Work out the finished part from the listing and answer in its coordinate system (mm). Face numbers are marked on the shaded views. A direction names the side the tool comes from. Coordinates: 2 decimals unless noted, no trailing zeros. Order: outer loops, then holes, each group sorted by start corner. A loop starts at its lowest first (then second) coordinate and runs counter-clockwise, first axis right, second up. Notation, with made-up numbers: M 83,-1 L 97,-1 A19 cw 97,20 Z; hole C -17,-30.5 d11. An arc over 180 degrees is marked long. Use a Markdown table: item, result.
from build123d import *

# Parameters (mm, degrees)
F0_R     = 0.5
F1_DEPTH = 75
F2_DEPTH = 58


with BuildPart() as f1:
    # F0 (on Front) → F1 (new body)
    with BuildSketch(Plane.XZ):
        with BuildLine():
            ThreePointArc((0.820651, 1.615282), (0.216927, 0.905898), (0, 0))
            ThreePointArc((0, 0), (2, -2), (4, 0))
            ThreePointArc((4, 0), (2.905898, 1.783073), (0.820651, 1.615282))
        make_face()
        with Locations((2, 0)):
            Circle(F0_R, mode=Mode.SUBTRACT)
    extrude(amount=F1_DEPTH)

    # F0 (on Front) → F2 (join)
    with BuildSketch(Plane.XZ):
        with BuildLine():
            Line((0, 9.6), (0, 0))
            ThreePointArc((0, 0), (0.216927, 0.905898), (0.820651, 1.615282))
            Line((0.820651, 1.615282), (0.820651, 10.211033))
            Line((0.820651, 10.211033), (-5.284584, 16.147118))
            Line((-5.284584, 16.147118), (-9.5, 16.147118))
            Line((-9.5, 16.147118), (-9.5, 15.5))
            Line((-9.5, 15.5), (-6.118823, 15.5))
            Line((-6.118823, 15.5), (0, 9.6))
        make_face()
        with BuildLine():
            ThreePointArc((0.820651, 1.615282), (0.216927, 0.905898), (0, 0))
            ThreePointArc((0, 0), (2, -2), (4, 0))
            ThreePointArc((4, 0), (2.905898, 1.783073), (0.820651, 1.615282))
        make_face()
        with Locations((2, 0)):
            Circle(F0_R, mode=Mode.SUBTRACT)
    extrude(amount=F2_DEPTH)


solid = f1.part
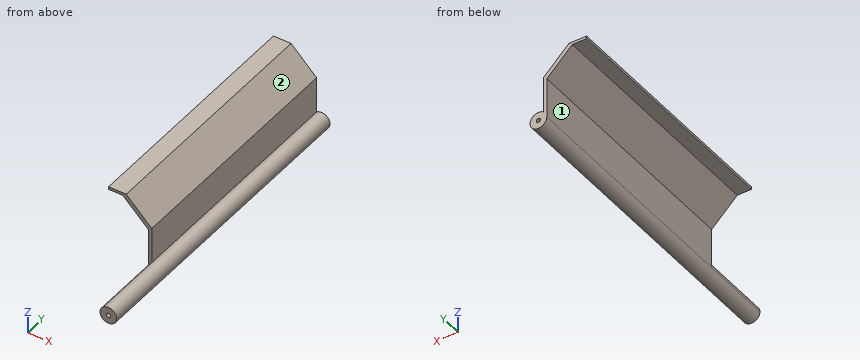
(1) Given P1, Ø2, axis at x = -1.5, y = -56.5, coming from the +Z side; P2, Ø1, axis at x = -6, y = -55.5, coming from the -Z side; P3, Ø1, axis at x = -7.5, y = -29, coming from the -Z side; P4, Ø6, axis at y = -62, z = 10, coming from the +X side, each flat-ended and moving along its own axis, determine where each tip first touches the part or whether it passes through.
Conclusion:
| item | result |
|---|---|
| P1 | z = 13.44 |
| P2 | z = 14.9 |
| P3 | z = 15.5 |
| P4 | through |
(2) A cutting plane is placed at A-A (y = -40). Determine the outline of the cut face in (x, z), then the cut area to 3 significant figures.
Conclusion:
| item | result |
|---|---|
| outline | M -9.5,15.5 L -6.12,15.5 L 0,9.6 L 0,0 A2 ccw long 0.82,1.62 L 0.82,10.21 L -5.28,16.15 L -9.5,16.15 Z; hole C 2,0 d1 |
| area | 30.2 mm2 |
(3) Which of the six approach directions +Z, -Z, +X, -X, +Y, -Y give full straight-line access (tool end or side, diameter ignored) to the marked faces 1 and 2?
Conclusion:
| item | result |
|---|---|
| face 1 | -Z, -X, +Y, -Y |
| face 2 | +Z, +X, +Y, -Y |
(4) Straight lines are drawn through the part: L1, parallel to Z at x = 2, y = -29.5; L2, parallel to Z at x = -8, y = -15.5; L3, parallel to X at y = -7, z = 6.5. For each, find the intervals that lie inside material, in ascending order.
Conclusion:
| item | result |
|---|---|
| L1 | -2 to -0.5, 0.5 to 2 |
| L2 | 15.5 to 16.15 |
| L3 | 0 to 0.82 |
(5) A cutting plane is placed at D-D (y = -67). Determine the outline of the cut face in (x, z).
Conclusion:
| item | result |
|---|---|
| outline | M 0,0 A2 ccw long 0.82,1.62 A2 ccw Z; hole C 2,0 d1 |
(6) A cutting plane is placed at B-B (x = -8.5). Determine the outline of the cut face in (y, z).
Conclusion:
| item | result |
|---|---|
| outline | M -58,15.5 L 0,15.5 L 0,16.15 L -58,16.15 Z |
(7) A cutting plane is placed at C-C (z = 7.25). Determine the outline of the cut face in (x, y).
Conclusion:
| item | result |
|---|---|
| outline | M 0,-58 L 0.82,-58 L 0.82,0 L 0,0 Z |
